Geometry: final body of the model. Coordinates: model frame, mm. Face numbers are marked on the shaded views. Round coordinates to 2 decimals unless told otherwise and drop trailing zeros. Order: outer loops, then holes, each group sorted by start corner. A loop starts at its lowest first (then second) coordinate and runs counter-clockwise, first axis right, second up. Notation, with made-up numbers: (32, 48.25) - (59, 48.25) arc R14 cw to (59, 71.25) - close; hole circle Ø10 at (7.5, 38). An arc over 180 degrees is marked (long way). Put each result on its own line as item: value. Start each with the question number.
(1) Section D-D (x = 38.5). Output: boundary loops of the cut face in (y, z).
(2) Section A-A (z = 25). Output: boundary loops of the cut face in (x, y).
(3) Pin query (flat end, axial travel): P1, Ø1.1, axis at x = -36, y = -20, coming from the +Z side; P2, Ø12, axis at x = 33, z = -0.5, coming from the -Y side; P3, Ø1.9, axis at x = -39, y = -20, coming from the -Z side; P4, Ø5.5, axis at y = -11.5, z = 27, coming from the -X side. Return the tip coordinate at first contact, or that it passes through.
(4) Material intervals for L1, parallel to Z at x = 0, y = -4.9 (3 decimals); L2, parallel to X at y = -5.5, z = 27; L3, parallel to Y at x = 38.5, z = -34, sorted ascending. Write a range as [from, to].
(5) Section B-B (y = -12.25). Output: boundary loops of the cut face in (x, z).
(6) Pull-direction query (Z, two-part tool) for the marked faces 1, 2 and 3; classes: released by +Z, released by -Z, zero draft, split by the parting line, or undercut.
(7) Section C-C (z = 34). Output: boundary loops of the cut face in (x, y), and give its area (3 significant figures).
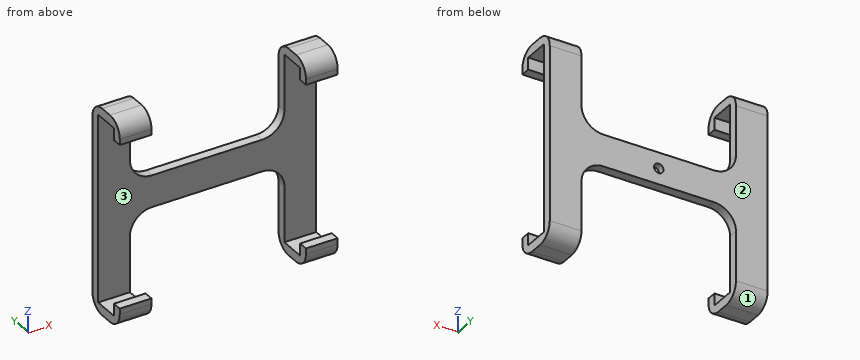
from build123d import *

# Parameters (mm, degrees)
F1_DEPTH      = 43.6245
F1_DEPTH_BACK = 43.6245
F2_R          = 1.905
F3_DEPTH      = 2.794
F5_DEPTH      = 25.4


# Not quite as in the source:
# - a length typed as a fraction of an inch, garbled in the dataset ("3 / 203.2 mm" for 3/8 in), is restored


with BuildPart() as f1:
    # F0 (on Right) → F1 (new body, two sides)
    with BuildSketch(Plane.YZ) as f1_sk:
        with BuildLine():
            Line((-8.008403407, 37.52215), (-8.008403407, 0))
            Line((-8.008403407, 0), (-8.008403407, -37.52215))
            Line((-8.008403407, -37.52215), (-18.168403407, -37.52215))
            Line((-18.168403407, -37.52215), (-18.168403407, -32.69615))
            Line((-18.168403407, -32.69615), (-21.978403407, -32.69615))
            Line((-21.978403407, -32.69615), (-21.978403407, -34.98215))
            ThreePointArc((-21.978403407, -34.98215), (-20.1185314675, -39.4722780605), (-15.628403407, -41.33215))
            Line((-15.628403407, -41.33215), (-10.548403407, -41.33215))
            ThreePointArc((-10.548403407, -41.33215), (-6.0582753465, -39.4722780605), (-4.198403407, -34.98215))
            Line((-4.198403407, -34.98215), (-4.198403407, 0))
            Line((-4.198403407, 0), (-4.198403407, 34.98215))
            ThreePointArc((-4.198403407, 34.98215), (-6.0582753465, 39.4722780605), (-10.548403407, 41.33215))
            Line((-10.548403407, 41.33215), (-15.628403407, 41.33215))
            ThreePointArc((-15.628403407, 41.33215), (-20.1185314675, 39.4722780605), (-21.978403407, 34.98215))
            Line((-21.978403407, 34.98215), (-21.978403407, 32.69615))
            Line((-21.978403407, 32.69615), (-18.168403407, 32.69615))
            Line((-18.168403407, 32.69615), (-18.168403407, 37.52215))
            Line((-18.168403407, 37.52215), (-8.008403407, 37.52215))
        make_face()
    extrude(amount=F1_DEPTH)
    extrude(f1_sk.sketch, amount=-F1_DEPTH_BACK)

    # F2 (on face) → F3 (cut)
    with BuildSketch(Plane(origin=(0, -4.198403407, 0), x_dir=(-1, 0, 0), z_dir=(0, 1, 0))):
        Circle(F2_R)
    extrude(amount=-F3_DEPTH, mode=Mode.SUBTRACT)

    # F4 (on face) → F5 (cut)
    with BuildSketch(Plane(origin=(0, -4.198403407, 0), x_dir=(-1, 0, 0), z_dir=(0, 1, 0))):
        with BuildLine():
            Line((-22.0345, 6.35), (22.0345, 6.35))
            ThreePointArc((22.0345, 6.35), (28.3206792847, 8.9538207153), (30.9245, 15.24))
            Line((30.9245, 15.24), (30.9245, 50.7227726401))
            Line((30.9245, 50.7227726401), (-30.9245, 50.7227726401))
            Line((-30.9245, 50.7227726401), (-30.9245, 15.24))
            ThreePointArc((-30.9245, 15.24), (-28.3206792847, 8.9538207153), (-22.0345, 6.35))
        make_face()
        with BuildLine():
            ThreePointArc((30.9245, -15.24), (28.3206792847, -8.9538207153), (22.0345, -6.35))
            Line((22.0345, -6.35), (-22.0345, -6.35))
            ThreePointArc((-22.0345, -6.35), (-28.3206792847, -8.9538207153), (-30.9245, -15.24))
            Line((-30.9245, -15.24), (-30.9245, -50.7227726401))
            Line((-30.9245, -50.7227726401), (30.9245, -50.7227726401))
            Line((30.9245, -50.7227726401), (30.9245, -15.24))
        make_face()
    extrude(amount=-F5_DEPTH, mode=Mode.SUBTRACT)


solid = f1.part
Checks:
1. outline: (-21.98, -34.98) arc R6.35 ccw to (-15.63, -41.33) - (-10.55, -41.33) arc R6.35 ccw to (-4.2, -34.98) - (-4.2, 34.98) arc R6.35 ccw to (-10.55, 41.33) - (-15.63, 41.33) arc R6.35 ccw to (-21.98, 34.98) - (-21.98, 32.7) - (-18.17, 32.7) - (-18.17, 37.52) - (-8.01, 37.52) - (-8.01, -37.52) - (-18.17, -37.52) - (-18.17, -32.7) - (-21.98, -32.7) - close
2. outline: (-43.62, -8.01) - (-30.92, -8.01) - (-30.92, -4.2) - (-43.62, -4.2) - close; (30.92, -8.01) - (43.62, -8.01) - (43.62, -4.2) - (30.92, -4.2) - close
3. P1: stops at z = 40.05
3. P2: stops at y = -8.01
3. P3: stops at z = -40.33
3. P4: passes through
4. L1: z = [-6.35, -1.905], [1.905, 6.35]
4. L2: x = [-43.62, -30.92], [30.92, 43.62]
4. L3: y = [-21.98, -18.17], [-8.01, -4.2]
5. outline: (-43.62, -41.33) - (-30.92, -41.33) - (-30.92, -37.52) - (-43.62, -37.52) - close; (-43.62, 37.52) - (-30.92, 37.52) - (-30.92, 41.33) - (-43.62, 41.33) - close; (30.92, -41.33) - (43.62, -41.33) - (43.62, -37.52) - (30.92, -37.52) - close; (30.92, 37.52) - (43.62, 37.52) - (43.62, 41.33) - (30.92, 41.33) - close
6. face 1: released by -Z
6. face 2: zero draft
6. face 3: undercut
7. outline: (-43.62, -21.98) - (-30.92, -21.98) - (-30.92, -18.17) - (-43.62, -18.17) - close; (-43.62, -8.01) - (-30.92, -8.01) - (-30.92, -4.2) - (-43.62, -4.2) - close; (30.92, -21.98) - (43.62, -21.98) - (43.62, -18.17) - (30.92, -18.17) - close; (30.92, -8.01) - (43.62, -8.01) - (43.62, -4.2) - (30.92, -4.2) - close
7. area: 194 mm²
